Check sheet for the modelled part. Datum: model origin and axes. Units: mm. Round coordinates to 2 decimals unless told otherwise and drop trailing zeros. Order: outer loops, then holes, each group sorted by start corner. A loop starts at its lowest first (then second) coordinate and runs counter-clockwise, first axis right, second up. Notation, with made-up numbers: (79.25, 79) -> (90.25, 79) arc R28 ccw to (90.25, 108) -> close; hole circle Ø1 at (28.25, 34). An arc over 180 degrees is marked (long way). Answer in a Markdown table with one row per item. Add a question column.
1. Material ranges on L1, parallel to X at y = 6.5, z = 0.05; L2, parallel to Y at x = 12, z = 0.05; L3, parallel to Y at x = 9.75, z = 0.05, recorded low to high. Write a range as from..to.
2. Sectioned sample at B-B, the plane x = 12.25. Record the boundary of the cut face in (y, z).
3. Sectioned sample at C-C, the plane y = 7. Record the boundary of the cut face in (x, z).
4. Sectioned sample at D-D, the plane x = 11.25. Record the boundary of the cut face in (y, z), then the cut area to 3 significant figures.
5. Sectioned sample at A-A, the plane z = 0.05. Record the boundary of the cut face in (x, y), then the cut area to 3 significant figures.
6. Depth check by flat-ended pin: P1, Ø2, axis at x = 13.5, y = 6.5, coming from the -Z side. Enter the tip coordinate at first touch or a pass-through.
```python
from build123d import *

# Parameters (mm, degrees)
SALIENTE_EXTRUIR1_DEPTH = 0.1


with BuildPart() as part:
    # Model → Saliente-Extruir1 (new body)
    with BuildSketch(Plane.XY):
        with BuildLine():
            ThreePointArc((5.820261238, 10.005409211), (9.186847838, 8.537831037), (12.859343802, 8.516280459))
            ThreePointArc((12.859343802, 8.516280459), (12.492089591, 7.026118334), (12.060688518, 5.553246333))
            ThreePointArc((12.060688518, 5.553246333), (12.413842974, 4.867805835), (12.894565351, 4.264935416))
            ThreePointArc((12.894565351, 4.264935416), (14.239685442, 2.677003657), (15.09298084, 0.778909273))
            ThreePointArc((15.09298084, 0.778909273), (14.77043638, -0.057438485), (14.107917756, -0.661244393))
            ThreePointArc((14.107917756, -0.661244393), (14.420283265, -1.49489014), (14.108158471, -2.328626043))
            ThreePointArc((14.108158471, -2.328626043), (10.869217247, -3.228854701), (7.514520421, -3.011688639))
            ThreePointArc((7.514520421, -3.011688639), (6.375365831, -2.483549755), (5.846898055, -1.344547705))
            ThreePointArc((5.846898055, -1.344547705), (6.252533801, 1.79168345), (6.779728877, 4.909784085))
            ThreePointArc((6.779728877, 4.909784085), (6.186082282, 7.436147735), (5.820261238, 10.005409211))
        make_face()
    extrude(amount=SALIENTE_EXTRUIR1_DEPTH)


solid = part.part
```
Answer key:
| question | item | result |
|---|---|---|
| 1 | L1 | x = 6.38..12.35 |
| 1 | L2 | y = -3.05..8.39 |
| 1 | L3 | y = -3.28..8.44 |
| 2 | outline | (-2.99, 0) -> (5.15, 0) -> (5.15, 0.1) -> (-2.99, 0.1) -> close; (6.17, 0) -> (8.42, 0) -> (8.42, 0.1) -> (6.17, 0.1) -> close |
| 3 | outline | (6.27, 0) -> (12.49, 0) -> (12.49, 0.1) -> (6.27, 0.1) -> close |
| 4 | outline | (-3.18, 0) -> (8.34, 0) -> (8.34, 0.1) -> (-3.18, 0.1) -> close |
| 4 | area | 1.15 mm² |
| 5 | outline | (5.82, 10.01) arc R29.05 ccw to (6.78, 4.91) arc R81.37 ccw to (5.85, -1.34) arc R1.83 ccw to (7.51, -3.01) arc R10.06 ccw to (14.11, -2.33) arc R1.27 ccw to (14.11, -0.66) arc R1.95 ccw to (15.09, 0.78) arc R7.45 ccw to (12.89, 4.26) arc R3.91 cw to (12.06, 5.55) arc R35.45 ccw to (12.86, 8.52) arc R9.13 cw to start |
| 5 | area | 86.6 mm² |
| 6 | P1 | passes through |
